Can you work these out from the model? Positions are in its coordinate system, mm. A direction names the side the tool comes from. Give positions to 0.01 mm unless a question says otherwise; leave off trailing zeros. Loops run counter-clockwise (first coordinate to the right, second up) from the corner with the lowest first, then second, coordinate; pieces in that order, holes last. Notation, with made-up numbers: (28, 10.25) - (56, 10.25) arc R4 ccw to (56, 17.25) - close; hole circle Ø9 at (10.5, 53.25). An arc over 180 degrees is marked (long way). Answer as a JSON object with one key per item and string values.
```python
from build123d import *

# Parameters (mm, degrees)
CUT_EXTRUDE_1_DEPTH = 3
FILLET_1_R          = 1
CHAMFER_1_SIZE      = 0.5


with BuildPart() as part:
    # 草图1 → 旋转1 (revolve)
    with BuildSketch(Plane.XY):
        Polygon((0, 0), (0, 5), (4.5, 5), (4.5, 3), (12.5, 3), (12.5, 2.5), (22.5, 2.5), (22.5, 0), align=None)
    revolve(axis=Axis((0, 0, 0), (1, 0, 0)))

    # 草图2 → 切除-拉伸1 (cut)
    with BuildSketch(Plane.ZY):
        Polygon((0, 1.732050808), (-1.5, 0.866025404), (-1.5, -0.866025404), (0, -1.732050808), (1.5, -0.866025404), (1.5, 0.866025404), align=None)
    extrude(amount=-CUT_EXTRUDE_1_DEPTH, mode=Mode.SUBTRACT)

    # 圆角1
    fillet_1_edges = [part.edges().sort_by_distance(p)[0] for p in [
        (0, -5, 0),
    ]]
    fillet(fillet_1_edges, radius=FILLET_1_R)

    # 倒角1
    chamfer_1_edges = [part.edges().sort_by_distance(p)[0] for p in [
        (22.5, -2.5, 0),
    ]]
    chamfer(chamfer_1_edges, length=CHAMFER_1_SIZE)


solid = part.part
```
1) I need wall thicknesses on L1, parallel to X at y = 3, z = 1.75; L2, parallel to Z at x = 20.25, y = 1.5; L3, parallel to Z at x = 13, y = 2. Which ranges of each line are inside material? Lowest first, please.
Check sheet entries:
{"L1": "0 to 4.5", "L2": "-2 to 2", "L3": "-1.5 to 1.5"}
2) Imagine slicing it at D-D on x = 16. Write out the boundary of the cut face in (y, z).
Check sheet entries:
{"outline": "circle Ø5 at (0, 0)"}
3) Imagine slicing it at A-A on x = 2.5. Write out the boundary of the cut face in (y, z), and give its area (3 significant figures).
Check sheet entries:
{"outline": "circle Ø10 at (0, 0); hole (-1.73, 0) - (-0.87, -1.5) - (0.87, -1.5) - (1.73, 0) - (0.87, 1.5) - (-0.87, 1.5) - close", "area": "70.7 mm2"}
4) Imagine slicing it at C-C on x = 9. Write out the boundary of the cut face in (y, z).
Check sheet entries:
{"outline": "circle Ø6 at (0, 0)"}
5) I'm going to push flat-ended pins straight in: P1, Ø6, axis at x = 13.5, y = -0.5, coming from the -Z side; P2, Ø4, axis at x = 18, y = 2, coming from the +Z side; P3, Ø1, axis at x = 11, z = 0.5, coming from the +Y side. Where does each tip first touch, or does it pass through?
Check sheet entries:
{"P1": "z = -3", "P2": "z = 2.5", "P3": "y = 3"}
6) If we mould it in two halves opening along Z, with no side actions, what happens to faces 4 (the flat face through (1.479, -1.293, -0.76)), 5 (the flat face through (4.5, 3.3, 0.1)), 6 (the cylindrical face through (9, -3, 0))? For each: released by +Z, released by -Z, zero draft, split by the parting line, or undercut.
Check sheet entries:
{"face 4": "undercut", "face 5": "zero draft", "face 6": "split by the parting line"}
7) Imagine slicing it at B-B on y = 0. Write out the boundary of the cut face in (x, z), and give its area (3 significant figures).
Check sheet entries:
{"outline": "(0, -4) arc R1 ccw to (1, -5) - (4.5, -5) - (4.5, -3) - (12.5, -3) - (12.5, -2.5) - (22, -2.5) - (22.5, -2) - (22.5, 2) - (22, 2.5) - (12.5, 2.5) - (12.5, 3) - (4.5, 3) - (4.5, 5) - (1, 5) arc R1 ccw to (0, 4) - (0, 1.5) - (3, 1.5) - (3, -1.5) - (0, -1.5) - close", "area": "133 mm2"}
8) Which directions (+Z, -Z, +X, -X, +Y, -Y) give clear straight access to the entire face, cutting with the end or side of a thin tool? Please do faces 1 (the cylindrical face through (17.32, -0.54, -2.44)), 2 (the flat face through (22.5, 0, 0)), 3 (the flat face through (1, 0, -1.5)).
Check sheet entries:
{"face 1": "+X", "face 2": "+Z, -Z, +X, +Y, -Y", "face 3": "-X"}
